Input: part model. Units: mm. Frame: model coordinates. Face numbers are marked on the shaded views. A direction names the side the tool comes from. Coordinates: 2 decimals unless noted, no trailing zeros. Write each loop counter-clockwise with the first axis right and the second up, starting at its lowest first coordinate (ties: lowest second). Pieces come first, ordered by that corner, then holes. Notation, with made-up numbers: M 37.25,88.25 L 44.25,88.25 A14 cw 44.25,114.25 Z; hole C 70.5,19 d4. An arc over 180 degrees is marked long. Write each question's results on one line, items separated by ' | '. Start each with the question number.
1. First-contact query: pin 1 (8 mm diameter, centred on x = 51, y = -4.5, fed in from -Z); pin 2 (2 mm diameter, centred on x = 44, y = 10, fed in from +Z); pin 3 (6.5 mm diameter, centred on x = 49.5, y = -0.5, fed in from +Z); pin 4 (2 mm diameter, centred on y = 21, z = 77.5, fed in from -X). Flat tips, straight axial feed; report the tip coordinate or a pass-through.
2. Ray query, probe 1 along Y at (x, z) = (48, 49); probe 2 along Z at (x, y) = (51.5, -18.5); probe 3 along X at (y, z) = (19, 42). Return the intervals inside material, ascending.
3. Section query C-C, the plane z = 55. Output: boundary loops of the cut face in (x, y).
4. Section query D-D, the plane z = 75. Count the separate pieces of the cut face and the enclosed holes in it, and give its area (3 significant figures).
5. Set-up query: the marked faces 1, 2 and 3. Return all of +Z, -Z, +X, -X, +Y, -Y with unobstructed straight access to the full face (end or side cutting, diameter ignored); none if empty.
6. Section query A-A, the plane y = 19.75. Output: boundary loops of the cut face in (x, z), and give its area (3 significant figures).
7. Section query B-B, the plane y = -27.5. Output: boundary loops of the cut face in (x, z).
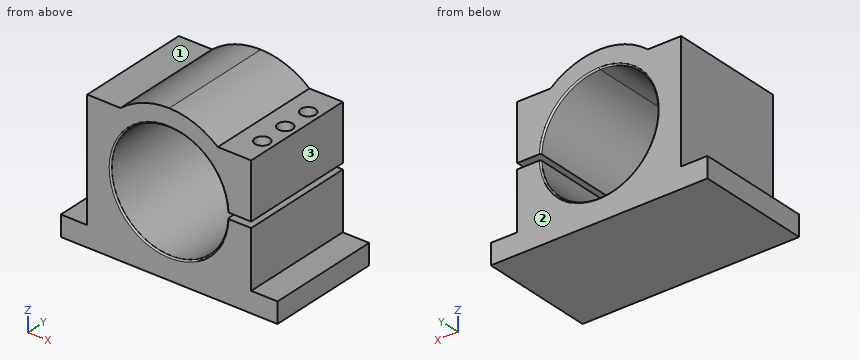
```python
from build123d import *

# Parameters (mm, degrees)
SKETCH1_W           = 148
SKETCH1_H           = 79
BOSS_EXTRUDE1_DEPTH = 14
SKETCH2_W           = 112
SKETCH2_H           = 79
BOSS_EXTRUDE2_DEPTH = 93
SKETCH3_R           = 40
CUT_EXTRUDE1_DEPTH  = 80
CUT_EXTRUDE2_DEPTH  = 80
CUT_EXTRUDE4_DEPTH  = 80
SKETCH9_R           = 3
CUT_EXTRUDE5_DEPTH  = 60
SKETCH10_R          = 5
CUT_EXTRUDE6_DEPTH  = 10
FILLET1_R           = 1


with BuildPart() as part:
    # Sketch1 → Boss-Extrude1 (new body)
    with BuildSketch(Plane.XY):
        Rectangle(SKETCH1_W, SKETCH1_H)
    extrude(amount=BOSS_EXTRUDE1_DEPTH)

    # Sketch2 → Boss-Extrude2 (add)
    with BuildSketch(Plane.XY.offset(14)):
        Rectangle(SKETCH2_W, SKETCH2_H)
    extrude(amount=BOSS_EXTRUDE2_DEPTH)

    # Sketch3 → Cut-Extrude1 (cut)
    with BuildSketch(Plane(origin=(0, 39.5, 0), x_dir=(1, 0, 0), z_dir=(0, 1, 0))):
        with Locations(Location((0, -55, 0), (0, 0, 270))):
            Circle(SKETCH3_R)
    extrude(amount=-CUT_EXTRUDE1_DEPTH, mode=Mode.SUBTRACT)

    # Sketch6 → Cut-Extrude2 (cut)
    with BuildSketch(Plane(origin=(0, 39.5, 0), x_dir=(1, 0, 0), z_dir=(0, 1, 0))):
        with BuildLine():
            ThreePointArc((0, -107), (-17.663521733, -103.908077043), (-33.226495452, -95))
            Line((-33.226495452, -95), (-56, -95))
            Line((-56, -95), (-56, -107))
            Line((-56, -107), (0, -107))
        make_face()
        with BuildLine():
            ThreePointArc((33.226495452, -95), (17.663521733, -103.908077043), (0, -107))
            Line((0, -107), (56, -107))
            Line((56, -107), (56, -95))
            Line((56, -95), (33.226495452, -95))
        make_face()
    extrude(amount=-CUT_EXTRUDE2_DEPTH, mode=Mode.SUBTRACT)

    # Sketch8 → Cut-Extrude4 (cut)
    with BuildSketch(Plane(origin=(0, 39.5, 0), x_dir=(1, 0, 0), z_dir=(0, 1, 0))):
        Polygon((56, -55), (56, -57), (38.221026174, -57), (38.221026174, -53), (56, -53), align=None)
    extrude(amount=-CUT_EXTRUDE4_DEPTH, mode=Mode.SUBTRACT)

    # Sketch9 → Cut-Extrude5 (cut)
    with BuildSketch(Plane.XY.offset(95)):
        with Locations((48, 19.75)):
            Circle(SKETCH9_R)
        with Locations((48, 0)):
            Circle(SKETCH9_R)
        with Locations((48, -19.75)):
            Circle(SKETCH9_R)
    extrude(amount=-CUT_EXTRUDE5_DEPTH, mode=Mode.SUBTRACT)

    # Sketch10 → Cut-Extrude6 (cut)
    with BuildSketch(Plane.XY.offset(95)):
        with Locations((48, 19.75)):
            Circle(SKETCH10_R)
        with Locations((48, 0)):
            Circle(SKETCH10_R)
        with Locations((48, -19.75)):
            Circle(SKETCH10_R)
    extrude(amount=-CUT_EXTRUDE6_DEPTH, mode=Mode.SUBTRACT)

    # Fillet1
    fillet1_edges = [part.edges().sort_by_distance(p)[0] for p in [
        (-28.982753492, 39.5, 27.431902496),
        (-28.982753492, -39.5, 27.431902496),
    ]]
    fillet(fillet1_edges, radius=FILLET1_R)


solid = part.part
```
Answer:
1) pin 1: z = 0 | pin 2: z = 95 | pin 3: z = 85 | pin 4: x = -56
2) probe 1: -39.5 to -22.75, -16.75 to -3, 3 to 16.75, 22.75 to 39.5 | probe 2: 0 to 53, 57 to 85 | probe 3: -56 to -37.83, 37.83 to 45.1, 50.9 to 56
3) outline: M -56,-39.5 L -41,-39.5 A1 ccw -40,-38.5 L -40,38.5 A1 ccw -41,39.5 L -56,39.5 Z
4) separate pieces: 2 | enclosed holes: 3 | area: 3,290 mm^2
5) face 1: +Z, -X, +Y, -Y | face 2: +Z, -Z, +X, -X, +Y | face 3: +Z, +X, +Y, -Y
6) outline: M -74,0 L 74,0 L 74,14 L 56,14 L 56,53 L 51,53 L 51,35 L 45,35 L 45,53 L 39.95,53 A40 cw long 39.95,57 L 45,57 L 45,85 L 43,85 L 43,95 L 33.23,95 A52 ccw -33.23,95 L -56,95 L -56,14 L -74,14 Z; M 51,57 L 56,57 L 56,95 L 53,95 L 53,85 L 51,85 Z | area: 6,220 mm^2
7) outline: M -74,0 L 74,0 L 74,14 L 56,14 L 56,53 L 39.95,53 A40 cw long 39.95,57 L 56,57 L 56,95 L 33.23,95 A52 ccw -33.23,95 L -56,95 L -56,14 L -74,14 Z
